Geometry: final body of the model. Coordinates: model frame, mm. A direction names the side the tool comes from. Give positions to 0.01 mm unless a question says otherwise; leave off trailing zeros. Write each loop counter-clockwise with the first axis right and the second up, starting at its lowest first coordinate (ties: lowest second). Pieces come first, ordered by that corner, then holes. Notation, with made-up numbers: M 82.25,3.25 L 129.25,3.25 A28 ccw 129.25,21.25 Z; hole C 65.5,17.5 d3. An arc over 180 degrees is marked long. Answer as a JSON object with one key per item and string values.
from build123d import *

# Parameters (mm, degrees)
F0_R     = 10.9982
F1_DEPTH = 6.35


with BuildPart() as f1:
    # F0 (on Top) → F1 (new body)
    with BuildSketch(Plane.XY):
        Polygon((-7.332348, -12.7), (7.332348, -12.7), (14.664697, -25.4), (29.329394, -25.4), (36.661742, -12.7), (29.329394, 0), (14.664697, 0), (7.332348, 12.7), (14.664697, 25.4), (7.332348, 38.1), (-7.332348, 38.1), (-14.664697, 25.4), (-7.332348, 12.7), (-14.664697, 0), (-29.690504, 0.625461), (-37.383962, -12.7), (-29.690504, -26.025461), (-14.303587, -26.025461), align=None)
        with Locations((-21.997045, -12.7)):
            Circle(F0_R, mode=Mode.SUBTRACT)
        with Locations((21.997045, -12.7)):
            Circle(F0_R, mode=Mode.SUBTRACT)
        Circle(F0_R, mode=Mode.SUBTRACT)
        with Locations((0, 25.4)):
            Circle(F0_R, mode=Mode.SUBTRACT)
    extrude(amount=-F1_DEPTH)


solid = f1.part
1) Set-up query: faces 1 (the flat face through (22, -25.4, -3)), 2 (the flat face through (11.05, 6.26, -3.13)), 3 (the flat face through (-11.05, 19.14, -3.13)), 4 (the flat face through (22, 0, -3)). Return all of +Z, -Z, +X, -X, +Y, -Y with unobstructed straight access to the full face (end or side cutting, diameter ignored); none if empty.
Geometry check:
{"face 1": "+Z, -Z, +X, -Y", "face 2": "+Z, -Z, +X", "face 3": "+Z, -Z, -X", "face 4": "+Z, -Z, +X, +Y"}
2) Line query: line 1 (Y direction, x = 0, z = -3); line 2 (Y direction, x = 7.5, z = -1.5); line 3 (Y direction, x = 12, z = -0.5). Output: solid intervals per line, ascending. Write a range as from..to.
Geometry check:
{"line 1": "y = -12.7..-11, 11..14.4, 36.4..38.1", "line 2": "y = -12.99..-8.04, 8.04..12.41, 12.99..17.36, 33.44..37.81", "line 3": "y = -20.78..-17.28, -8.12..4.62, 20.78..30.02"}
3) Contact query for flat-ended pins moving along their axis: P1, Ø3, axis at y = 16, z = -5.5, coming from the -X side; P2, Ø3, axis at y = 11.5, z = -1, coming from the +X side; P3, Ø17.5, axis at x = 0, y = 25.4, coming from the -Z side; P4, Ø3, axis at x = -2.5, z = -3, coming from the -Y side. Output: stop coordinate, or through.
Geometry check:
{"P1": "stops at x = -10.1", "P2": "stops at x = 8.89", "P3": "passes through", "P4": "stops at y = -12.7"}
4) Cut plane A-A on x = 0. Return loops of the section in (y, z).
Geometry check:
{"outline": "M -12.7,-6.35 L -11,-6.35 L -11,0 L -12.7,0 Z; M 11,-6.35 L 14.4,-6.35 L 14.4,0 L 11,0 Z; M 36.4,-6.35 L 38.1,-6.35 L 38.1,0 L 36.4,0 Z"}
5) Cut plane D-D on x = -17.5. Return loops of the section in (y, z), and give its area (3 significant figures).
Geometry check:
{"outline": "M -26.03,-6.35 L -22.74,-6.35 L -22.74,0 L -26.03,0 Z; M -2.66,-6.35 L 0.12,-6.35 L 0.12,0 L -2.66,0 Z", "area": "38.5 mm2"}
6) Cut plane C-C on y = 4.5. Return loops of the section in (x, z), and give its area (3 significant figures).
Geometry check:
{"outline": "M -12.07,-6.35 L -10.04,-6.35 L -10.04,0 L -12.07,0 Z; M 10.04,-6.35 L 12.07,-6.35 L 12.07,0 L 10.04,0 Z", "area": "25.8 mm2"}
7) Cut plane B-B on z = -1.75. Return loops of the section in (x, y).
Geometry check:
{"outline": "M -37.38,-12.7 L -29.69,-26.03 L -14.3,-26.03 L -7.33,-12.7 L 7.33,-12.7 L 14.66,-25.4 L 29.33,-25.4 L 36.66,-12.7 L 29.33,0 L 14.66,0 L 7.33,12.7 L 14.66,25.4 L 7.33,38.1 L -7.33,38.1 L -14.66,25.4 L -7.33,12.7 L -14.66,0 L -29.69,0.63 Z; hole C -22,-12.7 d22; hole C 0,0 d22; hole C 0,25.4 d22; hole C 22,-12.7 d22"}
8) Pull-direction query (X, two-part tool) for faces 5 (the cylindrical face through (-2.384, 14.663, -3.131)), 6 (the flat face through (10.947, -18.961, -3.131)), 7 (the flat face through (-12, -1, 0)), 8 (the flat face through (33.047, -6.439, -3.131)); classes: pulls with the +X half, pulls with the -X half, needs draft (parallel to the pull), parting line crosses it, or undercut.
Geometry check:
{"face 5": "undercut", "face 6": "undercut", "face 7": "needs draft", "face 8": "pulls with the +X half"}
